```python
from build123d import *

# Parameters (mm, degrees)
SKETCH1_R            = 15.8
SKETCH1_R_2          = 12.8
BOSS_EXTRUDE1_DEPTH  = 5
SKETCH2_W            = 5
SKETCH2_H            = 19.399038491
BOSS_EXTRUDE2_DEPTH  = 5
BOSS_EXTRUDE3_DEPTH  = 5
FILLET1_R            = 1
SKETCH38_W           = 12
SKETCH38_H           = 3.5
BOSS_EXTRUDE28_DEPTH = 12
CUT_EXTRUDE3_REACH   = 54.687
SKETCH39_R           = 2.75
CHAMFER1_SIZE        = 2.5
FILLET3_R            = 1
SKETCH1_3_R          = 12.8
SKETCH1_3_R_2        = 11.5
BOSS_EXTRUDE29_DEPTH = 1


with BuildPart() as part:
    # Sketch1 → Boss-Extrude1 (new body)
    with BuildSketch(Plane(origin=(0, 0, 0), x_dir=(0, 0, -1), z_dir=(1, 0, 0))):
        Circle(SKETCH1_R)
        Circle(SKETCH1_R_2, mode=Mode.SUBTRACT)
    extrude(amount=-BOSS_EXTRUDE1_DEPTH)

    # Sketch2 → Boss-Extrude2 (add)
    with BuildSketch(Plane(origin=(0, 0, 0), x_dir=(0, 0, -1), z_dir=(1, 0, 0))):
        with Locations((0, -25.300480755)):
            Rectangle(SKETCH2_W, SKETCH2_H)
    extrude(amount=-BOSS_EXTRUDE2_DEPTH)

    # Sketch3 → Boss-Extrude3 (add)
    with BuildSketch(Plane(origin=(0, 0, 0), x_dir=(0, 0, -1), z_dir=(1, 0, 0))):
        Polygon((-9.5, -35), (-9.5, -34), (9.5, -34), (9.5, -35), (3.05, -35), (3.05, -37.4), (5.45, -37.4), (5.45, -38.4), (3.05, -40), (-3.05, -40), (-5.45, -38.4), (-5.45, -37.4), (-3.05, -37.4), (-3.05, -35), align=None)
    extrude(amount=-BOSS_EXTRUDE3_DEPTH)

    # Fillet1
    fillet1_edges = [part.edges().sort_by_distance(p)[0] for p in [
        (0, -37.9, 5.45),
        (0, -37.9, -5.45),
    ]]
    fillet(fillet1_edges, radius=FILLET1_R)

    # Sketch38 → Boss-Extrude28 (add)
    with BuildSketch(Plane.ZY.offset(5)):
        with Locations((0, -33.25)):
            Rectangle(SKETCH38_W, SKETCH38_H)
    extrude(amount=BOSS_EXTRUDE28_DEPTH)

    # Sketch39 → Cut-Extrude3 (cut, up to next)
    with BuildSketch(Plane(origin=(0, -31.5, 0), x_dir=(1, 0, 0), z_dir=(0, 1, 0)), mode=Mode.PRIVATE) as cut_extrude3_sk1:
        with Locations(Location((-11, 0, 0), (0, 0, 270))):
            Circle(SKETCH39_R)
    cut_extrude3_tool1 = extrude(cut_extrude3_sk1.sketch, amount=-CUT_EXTRUDE3_REACH, mode=Mode.PRIVATE) & part.part
    add(cut_extrude3_tool1.solids().sort_by_distance((-11, -31.5, 0))[0], mode=Mode.SUBTRACT)

    # Chamfer1
    chamfer1_edges = [part.edges().sort_by_distance(p)[0] for p in [
        (-5, -31.5, 4.25),
        (-5, -31.5, -4.25),
    ]]
    chamfer(chamfer1_edges, length=CHAMFER1_SIZE - 0.0001)  # a hair under: the kernel refuses the full size

    # Fillet3
    fillet3_edges = [part.edges().sort_by_distance(p)[0] for p in [
        (-5, 0, 12.8),
    ]]
    fillet(fillet3_edges, radius=FILLET3_R)

    # Sketch1<3> → Boss-Extrude29 (add)
    with BuildSketch(Plane(origin=(0, 0, 0), x_dir=(0, 0, -1), z_dir=(1, 0, 0))):
        Circle(SKETCH1_3_R)
        Circle(SKETCH1_3_R_2, mode=Mode.SUBTRACT)
    extrude(amount=-BOSS_EXTRUDE29_DEPTH)


solid = part.part
```
CAD build for the part. Positions are in the model's coordinates, mm. A direction names the side the tool comes from. Coordinates: 2 decimals unless noted, no trailing zeros. Loops run counter-clockwise (first coordinate to the right, second up) from the corner with the lowest first, then second, coordinate; pieces in that order, holes last. Notation, with made-up numbers: (82.25, -7.75) - (102.25, -7.75) arc R19 ccw to (102.25, 21.25) - close; hole circle Ø4 at (-27.5, 61.25). An arc over 180 degrees is marked (long way). Use CSV: the item, a comma, the result in double quotes. Start each with the question number.
Q1. Cut at D-D, the plane y = -20. List the corners of the cut face in (x, z).
Q2. Cut at C-C, the plane x = -11. List the corners of the cut face in (y, z).
Q3. Probe probe 1 along X at (y, z) = (-33.9, 0); probe 2 along Y at (x, z) = (-2.8, 0); probe 3 along Y at (x, z) = (-3.25, 9). List the from-to ranges inside material, lowest first. Write a range as from..to.
Q4. Drop flat-ended pins along their axis: P1, Ø6, axis at x = -3.5, z = 5.5, coming from the -Y side; P2, Ø6, axis at x = -9, z = 2.5, coming from the +Y side; P3, Ø1, axis at x = -13.5, y = -33, coming from the +Z side; P4, Ø6, axis at x = -2.5, y = -27, coming from the +Z side. Give the stop position or say it passes through.
Q5. Cut at A-A, the plane y = 0. List the corners of the cut face in (x, z), then the cut area to 3 significant figures.
Q6. Cut at B-B, the plane z = 0. List the corners of the cut face in (x, y), then the cut area to 3 significant figures.
Q7. 3-axis set-ups, long thin cutter, end or side, ignore diameter. For faces 1 (the flat face through (-11, -33, 6)), 2 (the flat face through (-2.5, -34.5, 9.5)), 3 (the flat face through (-2, -36, -3.05)): which of +Z, -Z, +X, -X, +Y, -Y reach the whole face in a straight line?
Q8. Two-plate mould, pull along Y, no slides. Class faces 4 (the flat face through (-2, -34, -6)), 5 (the flat face through (-2.5, -34.5, -9.5)), 6 (the flat face through (-2.465, -39.211, 4.233)): +Y half, -Y half, draft (parallel to the pull), parting line (faces both ways), or undercut.
Here are the results:
1,outline,"(-5, -2.5) - (0, -2.5) - (0, 2.5) - (-5, 2.5) - close"
2,outline,"(-35, -6) - (-31.5, -6) - (-31.5, -2.75) - (-35, -2.75) - close; (-35, 2.75) - (-31.5, 2.75) - (-31.5, 6) - (-35, 6) - close"
3,probe 1,"-17..-13.75, -8.25..0"
3,probe 2,"-40..-12.8, 12.8..15.8"
3,probe 3,"-35..-34, -12.99..-9.1, 9.1..12.99"
4,P1,"y = -40"
4,P2,"y = -31.5"
4,P3,"z = 6"
4,P4,"z = 2.5"
5,outline,"(-5, -15.8) - (0, -15.8) - (0, -11.5) - (-1, -11.5) - (-1, -12.8) - (-4, -12.8) arc R1 ccw to (-5, -13.8) - close; (-5, 13.8) arc R1 ccw to (-4, 12.8) - (-1, 12.8) - (-1, 11.5) - (0, 11.5) - (0, 15.8) - (-5, 15.8) - close"
5,area,"32.2 mm2"
6,outline,"(-17, -35) - (-13.75, -35) - (-13.75, -31.5) - (-17, -31.5) - close; (-8.25, -35) - (-5, -35) - (-5, -40) - (0, -40) - (0, -11.5) - (-1, -11.5) - (-1, -12.8) - (-4, -12.8) arc R1 ccw to (-5, -13.8) - (-5, -31.5) - (-8.25, -31.5) - close; (-5, 13.8) arc R1 ccw to (-4, 12.8) - (-1, 12.8) - (-1, 11.5) - (0, 11.5) - (0, 15.8) - (-5, 15.8) - close"
6,area,"176 mm2"
7,face 1,"+Z, -X, +Y, -Y"
7,face 2,"+Z, +X, -X, -Y"
7,face 3,"-Z, +X, -X"
8,face 4,"undercut"
8,face 5,"draft"
8,face 6,"-Y half"
